Source: CAD feature listing. Evaluate the final solid. Frame: model axes, mm. Round coordinates to 2 decimals unless told otherwise and drop trailing zeros. Order: outer loops, then holes, each group sorted by start corner. A loop starts at its lowest first (then second) coordinate and runs counter-clockwise, first axis right, second up. Notation, with made-up numbers: (-27.75, 65) -> (-12.75, 65) arc R24 ccw to (-12.75, 98) -> close; hole circle Ø8 at (-8.5, 69). An arc over 180 degrees is marked (long way). Answer as CSV lines item,"result".
from build123d import *

# Parameters (mm, degrees)
SKETCH1_W           = 71.428571428
SKETCH1_H           = 3.175
SKETCH1_W_2         = 71.428571429
BOSS_EXTRUDE1_DEPTH = 3.175


with BuildPart() as part:
    # Sketch1 → Boss-Extrude1 (new body)
    with BuildSketch(Plane.XY):
        Polygon((50.899754495, -0.012509515), (122.328325923, -0.012509515), (122.328325923, 3.162490485), (193.756897352, 3.162490485), (193.756897352, -0.012509515), (265.185468781, -0.012509515), (265.185468781, 3.162490485), (336.614040209, 3.162490485), (336.614040209, -0.012509515), (408.042611638, -0.012509515), (408.042611638, 3.162490485), (479.471183066, 3.162490485), (479.471183066, 126.337490485), (408.042611638, 126.337490485), (408.042611638, 129.512490485), (479.471183066, 129.512490485), (479.471183066, 252.687490485), (408.042611638, 252.687490485), (408.042611638, 255.862490485), (479.471183066, 255.862490485), (479.471183066, 294.037490485), (166.471183066, 294.037490485), (-20.528816934, 294.037490485), (-70.528816934, 294.037490485), (-70.528816934, 255.862490485), (50.899754495, 255.862490485), (50.899754495, 252.687490485), (-70.528816934, 252.687490485), (-70.528816934, 129.512490485), (50.899754495, 129.512490485), (50.899754495, 126.337490485), (-70.528816934, 126.337490485), (-70.528816934, 3.162490485), (50.899754495, 3.162490485), align=None)
        with Locations((300.899754495, 127.924990485)):
            Rectangle(SKETCH1_W, SKETCH1_H, mode=Mode.SUBTRACT)
        with Locations((300.899754495, 254.274990485)):
            Rectangle(SKETCH1_W, SKETCH1_H, mode=Mode.SUBTRACT)
        with Locations((158.042611638, 127.924990485)):
            Rectangle(SKETCH1_W_2, SKETCH1_H, mode=Mode.SUBTRACT)
        with Locations((158.042611638, 254.274990485)):
            Rectangle(SKETCH1_W_2, SKETCH1_H, mode=Mode.SUBTRACT)
    extrude(amount=BOSS_EXTRUDE1_DEPTH)


solid = part.part
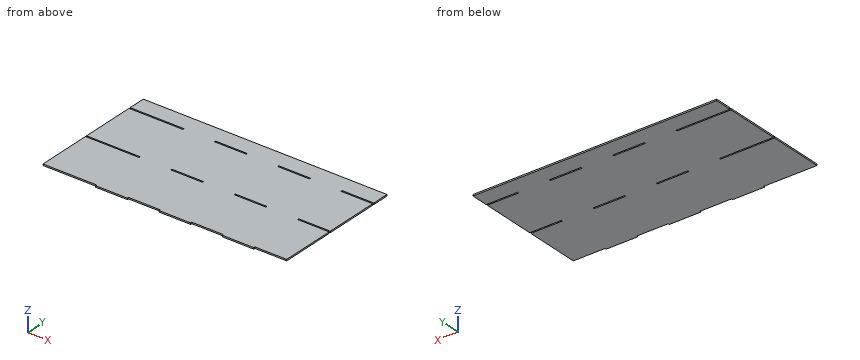
1. Section query A-A on x = 150.5. Return loops of the section in (y, z) (1 decimal).
Results below:
outline,"(3.2, 0) -> (126.3, 0) -> (126.3, 3.2) -> (3.2, 3.2) -> close; (129.5, 0) -> (252.7, 0) -> (252.7, 3.2) -> (129.5, 3.2) -> close; (255.9, 0) -> (294, 0) -> (294, 3.2) -> (255.9, 3.2) -> close"
2. Section query B-B on z = 1.25. Give the number of separate pieces and of enclosed holes in the cut face, and give its area (3 significant figures).
Results below:
separate pieces,"1"
enclosed holes,"4"
area,"159,000 mm2"
3. Line query: L1, parallel to Y at x = 130, z = 2.2. Output: solid intervals per line, ascending. Write a range as [from, to].
Results below:
L1,"[3.16, 126.34], [129.51, 252.69], [255.86, 294.04]"
4. Pin query (flat end, axial travel): pin 1 (1 mm diameter, centred on x = 166, z = 1, fed in from -Y); pin 2 (1 mm diameter, centred on y = 1, z = 2, fed in from -X). Return the tip coordinate at first contact, or that it passes through.
Results below:
pin 1,"y = 3.16"
pin 2,"x = 50.9"
